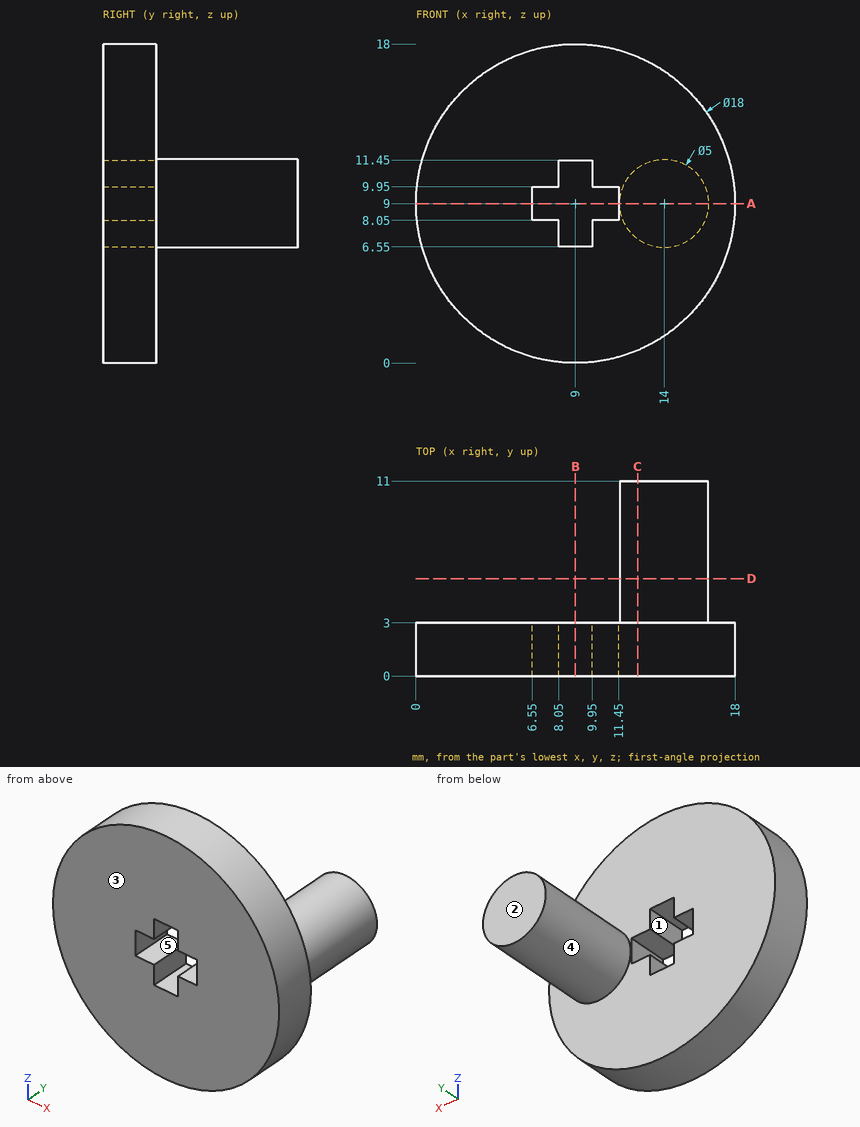
Answer from the drawing. Dimensions are ordinates in mm from the lowest x, y and z of the part. A direction names the side the tool comes from. Give positions to 0.01 mm unless a question says otherwise; leave off trailing zeros. Order: outer loops, then holes, each group sorted by start corner. A loop starts at its lowest first (then second) coordinate and runs counter-clockwise, first axis right, second up. Notation, with made-up numbers: (5, 71.5) -> (18, 71.5) arc R12 ccw to (18, 91.5) -> close; hole circle Ø3 at (55.25, 35). An arc over 180 degrees is marked (long way). One line per item, written item: value.
Item 1: Find section A-A, the plane z = 9. Give the vertices of the cut face in (x, y), plus the area to 3 significant figures.
Answer sheet:
outline: (0, 0) -> (6.55, 0) -> (6.55, 3) -> (0, 3) -> close; (11.45, 0) -> (18, 0) -> (18, 3) -> (16.5, 3) -> (16.5, 11) -> (11.5, 11) -> (11.5, 3) -> (11.45, 3) -> close
area: 79.3 mm²
Item 2: Determine the mould class of the marked faces 3, 4 and 5 for opening direction X: released by +X, released by -X, zero draft, split by the parting line, or undercut.
Answer sheet:
face 3: zero draft
face 4: split by the parting line
face 5: undercut
Item 3: A tool of negligible diameter and unlimited length cuts with its end or side. For the marked faces 1 and 2, from which of +Z, -Z, +X, -X, +Y, -Y can it reach the whole face along a straight path? Write none if from no direction.
Answer sheet:
face 1: +Y, -Y
face 2: +Z, -Z, +X, -X, +Y
Item 4: Find section C-C, the plane x = 12.5. Give the vertices of the cut face in (y, z), plus the area to 3 significant figures.
Answer sheet:
outline: (0, 0.71) -> (3, 0.71) -> (3, 7) -> (11, 7) -> (11, 11) -> (3, 11) -> (3, 17.29) -> (0, 17.29) -> close
area: 81.7 mm²
Item 5: Find section B-B, the plane x = 9. Give the vertices of the cut face in (y, z), plus the area to 3 significant figures.
Answer sheet:
outline: (0, 0) -> (3, 0) -> (3, 6.55) -> (0, 6.55) -> close; (0, 11.45) -> (3, 11.45) -> (3, 18) -> (0, 18) -> close
area: 39.3 mm²
Item 6: Find section D-D, the plane y = 5.5. Give the vertices of the cut face in (x, z), plus the area to 3 significant figures.
Answer sheet:
outline: circle Ø5 at (14, 9)
area: 19.6 mm²
Item 7: Straight lines are drawn through the part: probe 1 along X at (y, z) = (6, 9); probe 2 along Y at (x, z) = (7, 5); probe 3 along Z at (x, y) = (14, 7). For each, find the intervals that lie inside material, in ascending order.
Answer sheet:
probe 1: 11.5 to 16.5
probe 2: 0 to 3
probe 3: 6.5 to 11.5
Item 8: Flat-ended cylindrical pins translate along their axes: P1, Ø0.8, axis at x = 7.5, y = 1.5, coming from the -Z side; P2, Ø10, axis at x = 12, z = 7, coming from the +Y side; P3, Ø1.2, axis at y = 1, z = 11, coming from the -X side; P4, Ø1.2, axis at x = 10.5, y = 2, coming from the +Z side. Find the tip coordinate at first contact, or state that the pin passes through.
Answer sheet:
P1: z = 0.07
P2: y = 11
P3: x = 0.11
P4: z = 17.95
